Geometry check sheet. Reference: the model listing, model coordinates, mm. Round coordinates to 2 decimals unless told otherwise and drop trailing zeros. Loops run counter-clockwise (first coordinate to the right, second up) from the corner with the lowest first, then second, coordinate; pieces in that order, holes last. Notation, with made-up numbers: M 22.25,6.5 L 31.25,6.5 A14 cw 31.25,29.5 Z; hole C 73.25,-3 d5. An arc over 180 degrees is marked long. Use one line per item in the form item = value. Start each with the question number.
1. Material ranges on line 1 (Y direction, x = 0.5, z = 0.9); line 2 (X direction, y = 5.5, z = 0.2); line 3 (Y direction, x = -18, z = 3.5), recorded low to high.
2. Draft check along X on faces 1 (the flat face through (1.614, 8.5, 2.8)), 2 (the flat face through (15.056, 0, 3)). Enter one of: pulls with the +X half, pulls with the -X half, needs draft (parallel to the pull), parting line crosses it, or undercut.
3. Cross-section at C-C (z = 4.15). State how many separate pieces and enclosed holes the cut face has, then the cut area to 3 significant figures.
4. Cross-section at D-D (y = -9.5). Record the boundary of the cut face in (x, z), then the cut area to 3 significant figures.
5. Go/stop test with flat-tipped pins: pin 1 (1.5 mm diameter, centred on x = 8, y = -8.5, fed in from -Z); pin 2 (3 mm diameter, centred on x = 15.5, z = 2, fed in from +Y); pin 3 (1.3 mm diameter, centred on x = -17.5, z = 3, fed in from -Y); pin 4 (2 mm diameter, centred on y = -18, z = 3.5, fed in from +X). Record where each tip stops, or that it passes through.
6. Cross-section at B-B (y = -18). Record the boundary of the cut face in (x, z), then the cut area to 3 significant figures.
7. Cross-section at A-A (x = 0). Record the boundary of the cut face in (y, z).
```python
from build123d import *

# Parameters (mm, degrees)
F0_R     = 6.35
F1_DEPTH = 5.588


with BuildPart() as f1:
    # F0 (on Top) → F1 (new body)
    with BuildSketch(Plane.XY):
        Polygon((4.850337, 25.437864), (-4.228426, 25.437864), (-8.932546, 17.23641), (-6.893664, 13.286279), (-7.913105, 12.760089), (-10.211582, 16.488041), (-19.236901, 16.488041), (-23.656916, 8.629121), (-19.068447, 0.841377), (-14.800344, 0.841377), (-14.800344, -0.569267), (-19.068447, -0.569267), (-23.370794, -8.173046), (-19.047294, -15.802811), (-10.057353, -15.802811), (-7.992679, -12.275658), (-6.917777, -12.904869), (-8.919305, -16.324146), (-4.42692, -24.100309), (4.292383, -24.100309), (8.836989, -16.966333), (6.698302, -13.079478), (7.793717, -12.41559), (10.084728, -16.195757), (19.335584, -16.195757), (23.902084, -8.542322), (19.454879, -0.61194), (15.055753, -0.61194), (15.055753, 0.820334), (19.557185, 0.820334), (24.500479, 8.602312), (20.0502, 16.538178), (10.541808, 16.538178), (8.063308, 12.623042), (7.015632, 13.286279), (9.516286, 17.23641), align=None)
        Polygon((-2.673527, -12.323262), (2.558765, -12.41559), (4.9019, -16.281761), (2.347577, -20.372302), (-2.791393, -20.372302), (-5.113728, -16.231047), align=None, mode=Mode.SUBTRACT)
        Polygon((-19.284458, -7.828933), (-17.047726, -3.828624), (-12.058095, -3.828624), (-9.305194, -8.431129), (-11.584939, -12.173353), (-16.6606, -12.173353), align=None, mode=Mode.SUBTRACT)
        Polygon((-5.611179, -8.153478), (-6.985654, -5.693893), (-6.045224, -5.151337), (-4.569907, -7.708554), (-1.560098, -7.708554), (-1.560098, -8.659863), (-4.345217, -8.659863), (-5.783097, -11.016389), (-6.930758, -10.316121), align=None, mode=Mode.SUBTRACT)
        Polygon((-9.927894, 0.740779), (-8.559196, 3.295684), (-7.493752, 2.658462), (-9.08373, 0), (-7.612971, -2.58519), (-8.378716, -3.115653), (-9.801803, -0.577965), (-12.786955, -0.577965), (-12.786955, 0.740779), align=None, mode=Mode.SUBTRACT)
        Circle(F0_R, mode=Mode.SUBTRACT)
        Polygon((1.425454, -8.659863), (1.425454, -7.708554), (4.64753, -7.708554), (6.123088, -5.345567), (6.811032, -5.775151), (5.39455, -8.043533), (6.744049, -10.426221), (5.563155, -11.095052), (4.183921, -8.659863), align=None, mode=Mode.SUBTRACT)
        Polygon((9.052756, 0), (7.676018, 2.54796), (8.430281, 2.977073), (9.709381, 0.728767), (12.740129, 0.728767), (12.740129, -0.674656), (9.850005, -0.674656), (8.359578, -3.166668), (7.47518, -2.637726), align=None, mode=Mode.SUBTRACT)
        Polygon((11.511659, -12.436375), (9.375006, -8.634387), (12.20293, -4.046865), (17.041823, -4.046865), (19.272742, -8.131645), (16.601923, -12.436375), align=None, mode=Mode.SUBTRACT)
        Polygon((-19.42525, 8.33735), (-16.867618, 12.966663), (-11.931389, 12.966663), (-9.373757, 8.567536), (-12.05927, 3.887071), (-16.790888, 3.887071), align=None, mode=Mode.SUBTRACT)
        Polygon((-5.531086, 8.437562), (-6.984751, 10.933847), (-5.800158, 11.545281), (-4.429846, 9.078498), (-1.478518, 9.113127), (-1.46454, 7.921814), (-4.370745, 7.887715), (-5.950622, 5.246141), (-7.047472, 5.902147), align=None, mode=Mode.SUBTRACT)
        Polygon((-5.042579, 17.007749), (-2.5361, 21.381299), (2.933688, 21.445477), (5.290253, 16.879867), (2.962808, 12.760089), (-2.587253, 12.760089), align=None, mode=Mode.SUBTRACT)
        Polygon((1.614482, 7.921814), (1.614482, 9.113127), (4.530643, 9.113127), (5.981318, 11.518419), (6.998032, 10.905221), (5.379989, 8.222425), (6.919887, 5.724828), (6.216966, 5.291441), (4.595204, 7.921814), align=None, mode=Mode.SUBTRACT)
        Polygon((9.657924, 8.519574), (12.368077, 13.074742), (17.150848, 13.074742), (19.771752, 8.401072), (16.902813, 3.869183), (12.265772, 3.869183), align=None, mode=Mode.SUBTRACT)
    extrude(amount=F1_DEPTH)


solid = f1.part
```
Reported:
q1.line_1 = -24.1 to -20.37, -12.38 to -6.33, 6.33 to 12.76, 21.42 to 25.44
q1.line_2 = -21.81 to -17.75, -11.13 to -6.38, -5.8 to -3.17, 3.17 to 6.09, 6.56 to 11.35, 17.94 to 22.53
q1.line_3 = -15.8 to -9.96, -5.53 to -0.57, 0.84 to 5.93, 10.92 to 16.49
q2.face_1 = undercut
q2.face_2 = pulls with the +X half
q3.separate_pieces = 1
q3.enclosed_holes = 13
q3.area = 1,020 mm²
q4.outline = M -22.62,0 L -18.28,0 L -18.28,5.59 L -22.62,5.59 Z; M -9.96,0 L -6.43,0 L -6.43,5.59 L -9.96,5.59 Z; M -4.86,0 L 4.66,0 L 4.66,5.59 L -4.86,5.59 Z; M 6.22,0 L 9.86,0 L 9.86,5.59 L 6.22,5.59 Z; M 18.42,0 L 23.33,0 L 23.33,5.59 L 18.42,5.59 Z
q4.area = 145 mm²
q5.pin_1 = 0
q5.pin_2 = 16.54
q5.pin_3 = -15.8
q5.pin_4 = 8.82
q6.outline = M -7.95,0 L -4.12,0 L -4.12,5.59 L -7.95,5.59 Z; M 3.83,0 L 8.18,0 L 8.18,5.59 L 3.83,5.59 Z
q6.area = 45.7 mm²
q7.outline = M -24.1,0 L -20.37,0 L -20.37,5.59 L -24.1,5.59 Z; M -12.37,0 L -6.35,0 L -6.35,5.59 L -12.37,5.59 Z; M 6.35,0 L 12.76,0 L 12.76,5.59 L 6.35,5.59 Z; M 21.41,0 L 25.44,0 L 25.44,5.59 L 21.41,5.59 Z
